Check sheet for the modelled part. Datum: model origin and axes. Units: mm. A direction names the side the tool comes from. Round coordinates to 2 decimals unless told otherwise and drop trailing zeros. Loops run counter-clockwise (first coordinate to the right, second up) from the corner with the lowest first, then second, coordinate; pieces in that order, holes last. Notation, with made-up numbers: (54, 47.25) - (89, 47.25) arc R24 cw to (89, 61.25) - close; hole circle Ø8 at (22, -29.75). An arc over 180 degrees is marked (long way). Put each result on its own line as item: value. Start each with the question number.
Item 1: Tool access check on faces 1 (the flat face through (2, -9, -41.18)), 2 (the flat face through (-9, -17, 10.688)). Record the directions out of +Z, -Z, +X, -X, +Y, -Y that give a thin tool (end or side, any length) a straight path to the whole face; none if there is none.
Item 2: Material ranges on line 1 along Z through (x, y) = (-9, -16.75), recorded low to high.
Item 3: Section check A-A, the plane z = 5.5. Record the cut outline in (x, y).
Item 4: Section check B-B, the plane x = -7.5. Record the cut outline in (y, z), and give its area (3 significant figures).
Item 5: Draft check along X on faces 3 (the flat face through (2, -19.05, -10)), 4 (the flat face through (36.355, -9, -11)), 5 (the flat face through (-30.842, -9, -11)), 6 (the flat face through (-9, -17, -2.012)). Enter one of: pulls with the +X half, pulls with the -X half, needs draft (parallel to the pull), parting line crosses it, or undercut.
from build123d import *

# Parameters (mm, degrees)
F2_W     = 67.197241
F2_H     = 62.02823
F0_DEPTH = 19.05
F3_ANGLE = -180


with BuildPart() as f0:
    # F2 (on Front) → F0 (new body)
    with BuildSketch(Plane.XZ):
        with Locations((2.756816, -10.165736)):
            Rectangle(F2_W, F2_H)
    extrude(amount=F0_DEPTH)

    # F1 (on face) → F3 (revolve, cut)
    with BuildSketch(Plane.XZ.offset(19.05)):
        Polygon((-15.601805, -2.011621), (-9.251805, -2.011621), (-9.251805, 10.688379), (-12.426805, 10.688379), (-15.601805, 10.688379), (-15.601805, 8.631975), align=None)
    revolve(axis=Axis((-9.251805, -19.05, 4.338379), (0, 0, 1)), revolution_arc=F3_ANGLE, mode=Mode.SUBTRACT)


solid = f0.part
Check result:
1. face 1: -Z, +X, -X, +Y, -Y
1. face 2: -Y
2. line 1: -41.18 to -2.01, 10.69 to 20.85
3. outline: (-30.84, -19.05) - (-15.6, -19.05) arc R6.35 cw to (-2.9, -19.05) - (36.36, -19.05) - (36.36, 0) - (-30.84, 0) - close
4. outline: (-19.05, -41.18) - (0, -41.18) - (0, 20.85) - (-19.05, 20.85) - (-19.05, 10.69) - (-12.95, 10.69) - (-12.95, -2.01) - (-19.05, -2.01) - close
4. area: 1,100 mm²
5. face 3: needs draft
5. face 4: pulls with the +X half
5. face 5: pulls with the -X half
5. face 6: undercut
